CAD build for the part. Positions are in the model's coordinates, mm. Face numbers are marked on the shaded views. Coordinates: 2 decimals unless noted, no trailing zeros. Order: outer loops, then holes, each group sorted by start corner. A loop starts at its lowest first (then second) coordinate and runs counter-clockwise, first axis right, second up.
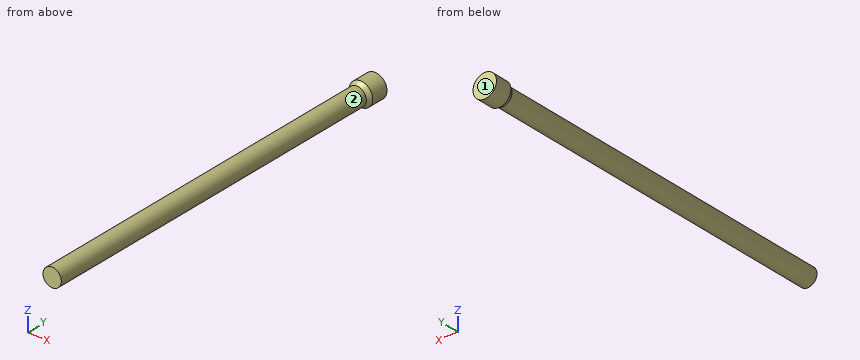
from build123d import *

# Parameters (mm, degrees)
SKETCH_1_R       = 2.5
EXTRUDE_1_DEPTH  = 2
SKETCH_2_R       = 1.95
EXTRUDE_2_DEPTH  = 80
CHAMFER_1_SIZE   = 1.5
CHAMFER_1_SIZE_2 = 2.598076211


with BuildPart() as part:
    # 草图1 → 凸台-拉伸1 (new body)
    with BuildSketch(Plane(origin=(0, 0, 0), x_dir=(1, 0, 0), z_dir=(0, 1, 0))):
        with Locations(Location((0, 0, 0), (0, 0, 270))):
            Circle(SKETCH_1_R)
    extrude(amount=EXTRUDE_1_DEPTH)

    # 草图2 → 凸台-拉伸2 (add)
    with BuildSketch(Plane.XZ):
        with Locations(Location((0, 0, 0), (0, 0, 270))):
            Circle(SKETCH_2_R)
    extrude(amount=EXTRUDE_2_DEPTH)

    # 倒角1
    # the kernel refuses this chamfer: 2.598076211, 1.5 mm, written as the material it adds along each edge
    with BuildSketch(Plane(origin=(0, 0, 0), x_dir=(0, 0, -1), z_dir=(-1, 0, 0))) as chamfer_1_piece_1_section:
        Polygon((1.95 + CHAMFER_1_SIZE, 0), (1.95, CHAMFER_1_SIZE_2), (1.95, 0), align=None)
    chamfer_1_piece_1 = revolve(axis=Axis((0, 0, 0), (0, -1, 0)), mode=Mode.PRIVATE)
    chamfer_1_piece_1 = chamfer_1_piece_1 & Plane(origin=(0, -2.153550613, 0), x_dir=(0, 0, 1), z_dir=(0, -1, 0)) * Cylinder(2.5, 14, mode=Mode.PRIVATE)
    add(chamfer_1_piece_1)


solid = part.part
1) Slice it at C-C (y = -47.5). List the corners of the cut face in (x, z).
2) Drill centre lines: probe 1 along Y at (x, z) = (-2.25, 0.55); probe 2 along Z at (x, y) = (0.2, -25). Where is each one in solid material? Low to high.
3) Pin check, flat tips, straight feed: P1, Ø1, axis at x = 0.5, y = -57, coming from the -Z side; P2, Ø2, axis at y = -67.5, z = 1, coming from the +X side; P3, Ø1, axis at y = -46.5, z = -1, coming from the -X side. Stop position of each tip, or through.
4) Slice it at B-B (z = 0). List the corners of the cut face in (x, y), plus the area to 3 significant figures.
5) Two-plate mould, pull along Y, no slides. Class the marked faces 1 and 2: released by +Y, released by -Y, zero draft, split by the parting line, or undercut.
6) Slice it at A-A (x = 0). List the corners of the cut face in (y, z).
Worked out:
1. outline: circle Ø3.9 at (0, 0)
2. probe 1: y = -1.96 to 2
2. probe 2: z = -1.94 to 1.94
3. P1: stops at z = -1.95
3. P2: stops at x = 1.95
3. P3: stops at x = -1.88
4. outline: (-2.5, -1.65) - (-1.95, -2.6) - (-1.95, -80) - (1.95, -80) - (1.95, -2.6) - (2.5, -1.65) - (2.5, 2) - (-2.5, 2) - close
4. area: 324 mm2
5. face 1: released by +Y
5. face 2: zero draft
6. outline: (-80, -1.95) - (-2.6, -1.95) - (-1.65, -2.5) - (2, -2.5) - (2, 2.5) - (-1.65, 2.5) - (-2.6, 1.95) - (-80, 1.95) - close
